from build123d import *

# Parameters (mm, degrees)
SKETCH2_W            = 42.6
SKETCH2_H            = 32
BOSS_EXTRUDE1_DEPTH  = 1.8
BOSS_EXTRUDE2_DEPTH  = 31.8
FILLET1_R            = 1
SKETCH4_W            = 1.505239861
SKETCH4_H            = 31.8
BOSS_EXTRUDE3_DEPTH  = 41
CUT_EXTRUDE1_DEPTH   = 41
SKETCH7_R            = 9.85
SKETCH7_R_2          = 4
BOSS_EXTRUDE4_DEPTH  = 4
FILLET1_OF_MIRROR2_R = 1
SKETCH8_R            = 12.15
BOSS_EXTRUDE5_DEPTH  = 5.4
SKETCH9_R            = 10.95
BOSS_EXTRUDE6_DEPTH  = 19
SKETCH11_R           = 12.15
BOSS_EXTRUDE7_DEPTH  = 5.2
SKETCH12_W           = 42.3
SKETCH12_H           = 25
BOSS_EXTRUDE8_DEPTH  = 1.8
SKETCH13_W           = 1.8
SKETCH13_H           = 25
BOSS_EXTRUDE9_DEPTH  = 44.3
CUT_EXTRUDE5_DEPTH   = 44.3
SKETCH18_R           = 9.85
SKETCH18_R_2         = 2.5
BOSS_EXTRUDE10_DEPTH = 4.2


with BuildPart() as part:
    # Sketch2 → Boss-Extrude1 (new body)
    with BuildSketch(Plane(origin=(0, 0, 0), x_dir=(1, 0, 0), z_dir=(0, 1, 0))):
        Rectangle(SKETCH2_W, SKETCH2_H)
    extrude(amount=BOSS_EXTRUDE1_DEPTH)

    # Sketch3 → Boss-Extrude2 (add)
    with BuildSketch(Plane.XY.offset(16)):
        Polygon((21.3, 1.8), (29.3, 14), (30.805239861, 14), (30.805239861, 13.012957468), (22.272152997, 0), (21.3, 0), align=None)
    boss_extrude2 = extrude(amount=-BOSS_EXTRUDE2_DEPTH)

    # Fillet1
    fillet1_edges = [part.edges().sort_by_distance(p)[0] for p in [
        (30.805239861, 13.012957468, 0.1),
        (22.272152997, 0, 0.1),
    ]]
    fillet(fillet1_edges, radius=FILLET1_R)

    # Sketch4 → Boss-Extrude3 (add)
    with BuildSketch(Plane(origin=(0, 14, 0), x_dir=(1, 0, 0), z_dir=(0, 1, 0))):
        with Locations((30.052619931, -0.1)):
            Rectangle(SKETCH4_W, SKETCH4_H)
    boss_extrude3 = extrude(amount=BOSS_EXTRUDE3_DEPTH)

    # Sketch5 → Cut-Extrude1 (cut)
    with BuildSketch(Plane(origin=(30.805239861, 0, 0), x_dir=(0, 0, -1), z_dir=(1, 0, 0))):
        with BuildLine():
            Line((-16, 55), (-16, 41.31158709))
            add(Edge.make_bspline(
                [(-0.1, 55), (-16, 55), (-16, 41.31158709)],
                knots=[1.570796327, 1.570796327, 1.570796327, 3.141592654, 3.141592654, 3.141592654], degree=2, weights=[1, 0.707106781, 1]))
            Line((-0.1, 55), (-16, 55))
        make_face()
        with BuildLine():
            Line((15.8, 55), (-0.1, 55))
            add(Edge.make_bspline(
                [(15.8, 41.31158709), (15.8, 55), (-0.1, 55)],
                knots=[0, 0, 0, 1.570796327, 1.570796327, 1.570796327], degree=2, weights=[1, 0.707106781, 1]))
            Line((15.8, 41.31158709), (15.8, 55))
        make_face()
    cut_extrude1 = extrude(amount=-CUT_EXTRUDE1_DEPTH, mode=Mode.SUBTRACT)

    # Sketch7 → Boss-Extrude4 (add)
    with BuildSketch(Plane.ZY.offset(-29.3)):
        with Locations((0.1, 41.31158709)):
            Circle(SKETCH7_R)
        with Locations((0.1, 41.31158709)):
            Circle(SKETCH7_R_2, mode=Mode.SUBTRACT)
    boss_extrude4 = extrude(amount=BOSS_EXTRUDE4_DEPTH)

    # Mirror2: Boss-Extrude2, Boss-Extrude3, Cut-Extrude1, Boss-Extrude4 across plane
    add(boss_extrude2.mirror(Plane(origin=(0, 0, 0), x_dir=(0, 0, 1), z_dir=(1, 0, 0))))
    add(boss_extrude3.mirror(Plane(origin=(0, 0, 0), x_dir=(0, 0, 1), z_dir=(1, 0, 0))))
    add(cut_extrude1.mirror(Plane(origin=(0, 0, 0), x_dir=(0, 0, 1), z_dir=(1, 0, 0))), mode=Mode.SUBTRACT)
    add(boss_extrude4.mirror(Plane(origin=(0, 0, 0), x_dir=(0, 0, 1), z_dir=(1, 0, 0))))

    # Fillet1 of Mirror2
    fillet1_of_mirror2_edges = [part.edges().sort_by_distance(p)[0] for p in [
        (-30.805239861, 13.012957468, 0.1),
        (-22.272152997, 0, 0.1),
    ]]
    fillet(fillet1_of_mirror2_edges, radius=FILLET1_OF_MIRROR2_R)

    # Sketch8 → Boss-Extrude5 (add)
    with BuildSketch(Plane.XZ):
        Circle(SKETCH8_R)
    extrude(amount=BOSS_EXTRUDE5_DEPTH)

    # Sketch9 → Boss-Extrude6 (add)
    with BuildSketch(Plane.XZ.offset(5.4)):
        Circle(SKETCH9_R)
    extrude(amount=BOSS_EXTRUDE6_DEPTH)

    # Sketch11 → Boss-Extrude7 (add)
    with BuildSketch(Plane.XZ.offset(24.4)):
        Circle(SKETCH11_R)
    extrude(amount=BOSS_EXTRUDE7_DEPTH)

    # Sketch12 → Boss-Extrude8 (add)
    with BuildSketch(Plane.XZ.offset(29.6)):
        Rectangle(SKETCH12_W, SKETCH12_H)
    extrude(amount=BOSS_EXTRUDE8_DEPTH)

    # Sketch13 → Boss-Extrude9 (add)
    with BuildSketch(Plane.XZ.offset(31.4)):
        with Locations((-20.25, 0)):
            Rectangle(SKETCH13_W, SKETCH13_H)
    boss_extrude9 = extrude(amount=BOSS_EXTRUDE9_DEPTH)

    # Sketch16 → Cut-Extrude5 (cut)
    with BuildSketch(Plane.ZY.offset(21.15)):
        with BuildLine():
            add(Edge.make_bspline(
                [(-12.5, -64.6), (-12.5, -75.7), (0, -75.7)],
                knots=[3.141592654, 3.141592654, 3.141592654, 4.71238898, 4.71238898, 4.71238898], degree=2, weights=[1, 0.707106781, 1]))
            Line((-12.5, -64.6), (-12.5, -75.7))
            Line((-12.5, -75.7), (3.5e-08, -75.7))
        make_face()
        with BuildLine():
            Line((12.5, -75.7), (12.5, -64.6))
            add(Edge.make_bspline(
                [(3.5e-08, -75.7), (12.5, -75.699999969), (12.5, -64.6)],
                knots=[4.712388984, 4.712388984, 4.712388984, 6.283185307, 6.283185307, 6.283185307], degree=2, weights=[0.999999999, 0.707106782, 1]))
            Line((3.5e-08, -75.7), (12.5, -75.7))
        make_face()
    cut_extrude5 = extrude(amount=-CUT_EXTRUDE5_DEPTH, mode=Mode.SUBTRACT)

    # Sketch18 → Boss-Extrude10 (add)
    with BuildSketch(Plane(origin=(-19.35, 0, 0), x_dir=(0, 0, -1), z_dir=(1, 0, 0))):
        with Locations((0, -58.4)):
            Circle(SKETCH18_R)
        with Locations((0, -58.4)):
            Circle(SKETCH18_R_2, mode=Mode.SUBTRACT)
    boss_extrude10 = extrude(amount=BOSS_EXTRUDE10_DEPTH)

    # Mirror3: Boss-Extrude9, Cut-Extrude5, Boss-Extrude10 across plane
    add(boss_extrude9.mirror(Plane(origin=(0, 0, 0), x_dir=(0, 0, 1), z_dir=(1, 0, 0))))
    add(cut_extrude5.mirror(Plane(origin=(0, 0, 0), x_dir=(0, 0, 1), z_dir=(1, 0, 0))), mode=Mode.SUBTRACT)
    add(boss_extrude10.mirror(Plane(origin=(0, 0, 0), x_dir=(0, 0, 1), z_dir=(1, 0, 0))))


solid = part.part
Build history of the part. All positions in model axes, mm. A direction names the side the tool comes from. Round coordinates to 2 decimals unless told otherwise and drop trailing zeros. Write each loop counter-clockwise with the first axis right and the second up, starting at its lowest first coordinate (ties: lowest second). Pieces come first, ordered by that corner, then holes. Notation, with made-up numbers: (39.25, 84) -> (60.25, 84) arc R29 cw to (60.25, 122) -> close; hole circle Ø2 at (86, -36). An arc over 180 degrees is marked (long way). Write item = value, one per line.
(1) Band-saw the part on A-A (y = -58.4). Give the cut face in (x, z).
Answer:
outline = (-21.15, -12.5) -> (-19.35, -12.5) -> (-19.35, -9.85) -> (-15.15, -9.85) -> (-15.15, -2.5) -> (-19.35, -2.5) -> (-19.35, 2.5) -> (-15.15, 2.5) -> (-15.15, 9.85) -> (-19.35, 9.85) -> (-19.35, 12.5) -> (-21.15, 12.5) -> close; (15.15, -9.85) -> (19.35, -9.85) -> (19.35, -12.5) -> (21.15, -12.5) -> (21.15, 12.5) -> (19.35, 12.5) -> (19.35, 9.85) -> (15.15, 9.85) -> (15.15, 2.5) -> (19.35, 2.5) -> (19.35, -2.5) -> (15.15, -2.5) -> close
(2) Band-saw the part on B-B (x = 0). Give the cut face in (y, z).
Answer:
outline = (-31.4, -12.5) -> (-29.6, -12.5) -> (-29.6, -12.15) -> (-24.4, -12.15) -> (-24.4, -10.95) -> (-5.4, -10.95) -> (-5.4, -12.15) -> (0, -12.15) -> (0, -16) -> (1.8, -16) -> (1.8, 16) -> (0, 16) -> (0, 12.15) -> (-5.4, 12.15) -> (-5.4, 10.95) -> (-24.4, 10.95) -> (-24.4, 12.15) -> (-29.6, 12.15) -> (-29.6, 12.5) -> (-31.4, 12.5) -> close
(3) Tool access for faces 4 (the face through (-25.24, 7.81, 0.32)), 5 (the face through (0, 1.8, 0)), 6 (the face through (-30.805, 34, 0)), 7 (the face through (-15.15, -60.5, -2.1)), 8 (the face through (19.35, -48, 0)): list every direction of +Z, -Z, +X, -X, +Y, -Y with a clear straight run to the whole face (end or side of a thin tool).
Answer:
face_4 = +Z, -Z
face_5 = +Z, -Z, +Y
face_6 = +Z, -Z, -X, +Y, -Y
face_7 = +Z, -Z, -Y
face_8 = none
(4) Probe L1, parallel to Y at x = 17, z = 0; L2, parallel to X at y = -58.5, z = -5; L3, parallel to X at y = 42, z = 1.5. List the from-to ranges inside material, lowest first.
Answer:
L1 = -68.25 to -60.9, -55.9 to -48.55, -31.4 to -29.6, 0 to 1.8
L2 = -21.15 to -15.15, 15.15 to 21.15
L3 = -30.81 to -29.3, 29.3 to 30.81
(5) Flat gauge pins, fed straight in: pin 1 (8 mm diameter, centred on y = -34.5, z = -6, fed in from -X); pin 2 (7.5 mm diameter, centred on x = -25, y = 17, fed in from -Z); pin 3 (4 mm diameter, centred on y = -57.5, z = 0.5, fed in from +X); pin 4 (12 mm diameter, centred on x = -5.5, y = -36, fed in from +Z). Where does each tip first touch, or does it go through?
Answer:
pin_1 = -21.15
pin_2 = through
pin_3 = 21.15
pin_4 = 12.5
(6) Two-plate mould, pull along X, no slides. Class faces 1 (the face through (-17.28, -56.29, -1.34)), 2 (the face through (-8.69, -14.77, -6.66)), 3 (the face through (-2, -5.4, 11)): pulls with the +X half, pulls with the -X half, needs draft (parallel to the pull), parting line crosses it, or undercut.
Answer:
face_1 = undercut
face_2 = parting line crosses it
face_3 = needs draft
